```python
from build123d import *


with BuildPart() as part:
    # Sketch1 → Revolve1 (revolve)
    with BuildSketch(Plane.XY, mode=Mode.PRIVATE) as revolve1_sk:
        Polygon((12.6365, 0.762), (12.6365, 62.738), (11.8745, 63.5), (0, 63.5), (0, 4.826), (6.1341, 4.826), (6.3881, 4.572), (6.3881, 0), (11.8745, 0), align=None)
    revolve(revolve1_sk.sketch.rotate(Axis((0, 0, 0), (0, 1, 0)), 90), axis=Axis((0, 0, 0), (0, 1, 0)))  # turned: the seam where the file's is

    # Sketch2 → Cut-Revolve1 (revolve, cut)
    with BuildSketch(Plane.XY, mode=Mode.PRIVATE) as cut_revolve1_sk:
        with BuildLine():
            Line((12.7, 43.307), (12.7, 42.545))
            Line((12.7, 42.545), (12.498605122, 42.746394878))
            ThreePointArc((12.498605122, 42.746394878), (12.424210245, 42.926), (12.498605122, 43.105605122))
            Line((12.498605122, 43.105605122), (12.7, 43.307))
        make_face()
    revolve(cut_revolve1_sk.sketch.rotate(Axis((0, 0, 0), (0, 1, 0)), 90), axis=Axis((0, 0, 0), (0, 1, 0)), mode=Mode.SUBTRACT)  # turned: the seam where the file's is


solid = part.part
```
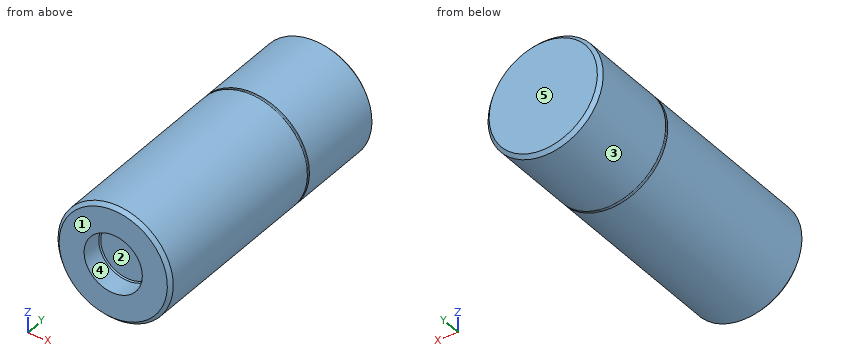
For this review, take the finished solid that the model builds, in its own axes (mm). Face numbers are marked on the shaded views. A direction names the side the tool comes from. Round coordinates to 2 decimals unless told otherwise and drop trailing zeros. Write each loop counter-clockwise with the first axis right and the second up, starting at its lowest first coordinate (ties: lowest second). Pieces come first, ordered by that corner, then holes. Notation, with made-up numbers: (21.25, -19) - (43.25, -19) arc R33 cw to (43.25, 12) - close; hole circle Ø4 at (-13, -32). An arc over 180 degrees is marked (long way). Use CSV: the item, a comma, the result in double quotes.
1) The part is to be moulded in two halves that separate along Z. For the marked faces 1, 2 and 3, say which applies: pulls with the +Z half, pulls with the -Z half, needs draft (parallel to the pull), parting line crosses it, or undercut.
Conclusion:
face 1,"needs draft"
face 2,"undercut"
face 3,"parting line crosses it"
2) Wall thickness on line 1 along X through (y, z) = (2.3, 0); line 2 along Y through (x, z) = (-1.25, 5); line 3 along Z through (x, y) = (3.5, 56): over which ranges is each line inside the solid? List them lowest first. Write a range as from..to.
Conclusion:
line 1,"x = -12.64..-6.39, 6.39..12.64"
line 2,"y = 4.83..63.5"
line 3,"z = -12.14..12.14"
3) Clearance check with flat-ended pins moving along their axes: pin 1 Ø8 at (y, z) = (48, -6) entering from -X; pin 2 Ø4 at (y, z) = (48, -9) entering from +X; pin 3 Ø1.5 at (y, z) = (17, 8) entering from +X; pin 4 Ø5 at (x, z) = (-8, -3) entering from -Y. State where each tip first meets the part, or that it passes through.
Conclusion:
pin 1,"stops at x = -12.48"
pin 2,"stops at x = 10.52"
pin 3,"stops at x = 10.35"
pin 4,"stops at y = 0"
4) Add section C-C on y = 49. Write out the cut boundary in (x, z).
Conclusion:
outline,"circle Ø25.27 at (0, 0)"
5) Add section A-A on x = 0. Write out the cut boundary in (y, z).
Conclusion:
outline,"(0, -11.87) - (0.76, -12.64) - (42.61, -12.64) - (42.75, -12.5) arc R0.25 cw to (43.11, -12.5) - (43.24, -12.64) - (62.74, -12.64) - (63.5, -11.87) - (63.5, 11.87) - (62.74, 12.64) - (43.24, 12.64) - (43.11, 12.5) arc R0.25 cw to (42.75, 12.5) - (42.61, 12.64) - (0.76, 12.64) - (0, 11.87) - (0, 6.39) - (4.57, 6.39) - (4.83, 6.13) - (4.83, -6.13) - (4.57, -6.39) - (0, -6.39) - close"
6) Add section B-B on z = 0. Write out the cut boundary in (x, y).
Conclusion:
outline,"(-12.64, 0.76) - (-11.87, 0) - (-6.39, 0) - (-6.39, 4.57) - (-6.13, 4.83) - (6.13, 4.83) - (6.39, 4.57) - (6.39, 0) - (11.87, 0) - (12.64, 0.76) - (12.64, 42.61) - (12.5, 42.75) arc R0.25 cw to (12.5, 43.11) - (12.64, 43.24) - (12.64, 62.74) - (11.87, 63.5) - (-11.87, 63.5) - (-12.64, 62.74) - (-12.64, 43.24) - (-12.5, 43.11) arc R0.25 cw to (-12.5, 42.75) - (-12.64, 42.61) - close"
7) For the marked faces 4 and 5, list the 3-axis set-ups (+Z, -Z, +X, -X, +Y, -Y) from which the entire face can be reached by the end or side of a thin tool; tool diameter is ignored.
Conclusion:
face 4,"-Y"
face 5,"+Z, -Z, +X, -X, +Y"
